from build123d import *

# Parameters (mm, degrees)
SKETCH1_W           = 24.4
SKETCH1_H           = 24.3
SKETCH1_W_2         = 20.4
SKETCH1_H_2         = 20.3
BOSS_EXTRUDE1_DEPTH = 40
SKETCH3_R           = 2.15
CUT_EXTRUDE1_DEPTH  = 40
CIRPATTERN1_COUNT   = 4


with BuildPart() as part:
    # Sketch1 → Boss-Extrude1 (new body)
    with BuildSketch(Plane(origin=(0, 0, 0), x_dir=(1, 0, 0), z_dir=(0, 1, 0))):
        Rectangle(SKETCH1_W, SKETCH1_H)
        Rectangle(SKETCH1_W_2, SKETCH1_H_2, mode=Mode.SUBTRACT)
    extrude(amount=BOSS_EXTRUDE1_DEPTH)

    # Sketch2 → Cut-Revolve1 (revolve, cut)
    with BuildSketch(Plane(origin=(0, 0, 0), x_dir=(0.7085572520498782, 0, -0.7056533288857395), z_dir=(0.7056533288857395, 0, 0.7085572520498782))):
        with BuildLine():
            Line((-19.218086421, 10), (-19.218086421, 30))
            ThreePointArc((-19.218086421, 30), (-17.218086421, 32), (-15.218086421, 30))
            Line((-15.218086421, 30), (-15.218086421, 10))
            ThreePointArc((-15.218086421, 10), (-17.218086421, 8), (-19.218086421, 10))
        make_face()
    revolve(axis=Axis((0.050102458, 40, -0.04989712), (-0.0012525594966950285, -0.9999984375102502, 0.0012474260561348032)), mode=Mode.SUBTRACT)

    # Sketch3 → Cut-Extrude1 (cut, symmetric)
    with BuildSketch(Plane.XY.offset(-10.15)):
        with Locations((0, 30)):
            Circle(SKETCH3_R)
        with Locations((0, 10)):
            Circle(SKETCH3_R)
    cut_extrude1 = extrude(amount=CUT_EXTRUDE1_DEPTH, both=True, mode=Mode.SUBTRACT)

    # CirPattern1: Cut-Extrude1 ×4 about axis
    cirpattern1_axis = Axis((0.050102458, 40, -0.04989712), (-0.0012525594966950285, -0.9999984375102502, 0.0012474260561348032))
    for i in range(1, CIRPATTERN1_COUNT):
        add(cut_extrude1.rotate(cirpattern1_axis, i * 360 / CIRPATTERN1_COUNT), mode=Mode.SUBTRACT)


solid = part.part
Read the model definition and answer for the solid it produces. Units are mm, in the model's axes. Coordinates: 2 decimals unless noted, no trailing zeros. Write each loop counter-clockwise with the first axis right and the second up, starting at its lowest first coordinate (ties: lowest second). Pieces come first, ordered by that corner, then holes. Notation, with made-up numbers: (56, 67) - (82, 67) arc R6 ccw to (82, 75) - close; hole circle Ø7 at (74.5, -17.75). An arc over 180 degrees is marked (long way). One line per question, with ' | ' between items.
Q1. Find section B-B, the plane z = 5. Write down the section's boundary in (x, y).
Result set:
outline: (-12.2, 0) - (-10.2, 0) - (-10.2, 40) - (-12.2, 40) - close; (10.2, 0) - (12.2, 0) - (12.2, 40) - (10.2, 40) - close
Q2. Consider L1, parallel to X at y = 24, z = -1.5; L2, parallel to Z at x = -5.25, y = 31.5; L3, parallel to X at y = 20, z = 9.5. Determine where each line is inside the solid, lowest interval first. Write a range as [from, to].
Result set:
L1: [-12.2, -10.2], [10.2, 12.2] | L2: [-12.15, -10.15], [10.15, 12.15] | L3: [-11.89, -10.2], [10.2, 11.94]
Q3. Find section A-A, the plane x = -8. Write down the section's boundary in (y, z).
Result set:
outline: (0, -12.15) - (40, -12.15) - (40, -10.15) - (0, -10.15) - close; (0, 10.15) - (40, 10.15) - (40, 12.15) - (0, 12.15) - close
Q4. This flat-tipped pin is pushed along its axis until it touches: P1, Ø6, axis at x = 3.5, z = 8.5, coming from the +Y side. Where does it stop, or does it pass through?
Result set:
P1: y = 40
Q5. Find section C-C, the plane x = 0. State how many separate pieces and enclosed holes the cut face has, plus the area to 3 significant figures.
Result set:
separate pieces: 6 | enclosed holes: 0 | area: 125 mm^2
Q6. Determine the mould class of faces 1 (the flat face through (-10.2, 20, 0)), 2 (the conical face through (10.85, 19.83, 10.72)) for opening direction Y: +Y half, -Y half, draft (parallel to the pull), parting line (faces both ways), or undercut.
Result set:
face 1: draft | face 2: undercut
